Source: CAD feature listing. Evaluate the final solid. Frame: model axes, mm. Coordinates: 2 decimals unless noted, no trailing zeros. Loops run counter-clockwise (first coordinate to the right, second up) from the corner with the lowest first, then second, coordinate; pieces in that order, holes last.
Item 1: Section query B-B, the plane x = -62. Return the cut outline in (y, z), then the cut area to 3 significant figures.
Item 2: Pull-direction query (X, two-part tool) for faces 1 (the cylindrical face through (-20.652, 1.521, 32.192)), 2 (the flat face through (-7, 3, 38)), 3 (the cylindrical face through (60.413, 1.521, 38.969)); classes: +X half, -X half, draft (parallel to the pull), parting line (faces both ways), or undercut.
Item 3: Pin query (flat end, axial travel): pin 1 Ø2 at (x, z) = (-19.5, 38) entering from -Y. Return the tip coordinate at first contact, or that it passes through.
Item 4: Line query: probe 1 along Z at (x, y) = (-97.5, 1.8); probe 2 along Z at (x, y) = (-44, 0.85); probe 3 along Z at (x, y) = (15, 2.35). Output: solid intervals per line, ascending.
Item 5: Section query A-A, the plane z = 20. Return the cut outline in (x, y), then the cut area to 3 significant figures.
Item 6: Section query C-C, the plane y = 1.4. State how many separate pieces and enclosed holes the cut face has, then the cut area to 3 significant figures.
```python
from build123d import *

# Parameters (mm, degrees)
SKETCH1_W           = 214
SKETCH1_H           = 186
BOSS_EXTRUDE1_DEPTH = 3
SKETCH2_R           = 23
SPEAKER_DEPTH       = 4
SKETCH4_R           = 3
SKETCH4_R_2         = 1.025
MOTOR_DEPTH         = 4
SKETCH6_W           = 6
SKETCH6_H           = 5
IZGARALAR_DEPTH     = 4
SKETCH7_R           = 9.5
MOTOR_KABLOSU_DEPTH = 4


with BuildPart() as part:
    # Sketch1 → Boss-Extrude1 (new body)
    with BuildSketch(Plane(origin=(0, 0, 0), x_dir=(1, 0, 0), z_dir=(0, 1, 0))):
        with Locations((-5.589552239, -39.100746269)):
            Rectangle(SKETCH1_W, SKETCH1_H)
    extrude(amount=BOSS_EXTRUDE1_DEPTH)

    # Sketch2 → Speaker (cut, through all)
    with BuildSketch(Plane(origin=(0, 3, 0), x_dir=(1, 0, 0), z_dir=(0, 1, 0))):
        with Locations((-42.589552239, -39.100746269)):
            Circle(SKETCH2_R)
    extrude(amount=-SPEAKER_DEPTH, mode=Mode.SUBTRACT)

    # Sketch4 → Motor (cut, through all)
    with BuildSketch(Plane(origin=(0, 3, 0), x_dir=(1, 0, 0), z_dir=(0, 1, 0))):
        with Locations((63.410447761, -39.100746269)):
            Circle(SKETCH4_R)
        with Locations((63.410447761, -31.100746269)):
            Circle(SKETCH4_R_2)
        with Locations((71.410447761, -39.100746269)):
            Circle(SKETCH4_R_2)
        with Locations((63.410447761, -47.100746269)):
            Circle(SKETCH4_R_2)
        with Locations((55.410447761, -39.100746269)):
            Circle(SKETCH4_R_2)
    extrude(amount=-MOTOR_DEPTH, mode=Mode.SUBTRACT)

    # Sketch6 → Izgaralar (cut, through all)
    with BuildSketch(Plane(origin=(0, 3, 0), x_dir=(1, 0, 0), z_dir=(0, 1, 0))):
        with Locations((-97.589552239, -122.600746269)):
            Rectangle(SKETCH6_W, SKETCH6_H)
        with Locations((-50.589552239, -122.600746269)):
            Rectangle(SKETCH6_W, SKETCH6_H)
        with Locations((-3.589552239, -122.600746269)):
            Rectangle(SKETCH6_W, SKETCH6_H)
        with Locations((-97.589552239, 44.399253731)):
            Rectangle(SKETCH6_W, SKETCH6_H)
        with Locations((-50.589552239, 44.399253731)):
            Rectangle(SKETCH6_W, SKETCH6_H)
        with Locations((-3.589552239, 44.399253731)):
            Rectangle(SKETCH6_W, SKETCH6_H)
        with Locations((43.410447761, -122.600746269)):
            Rectangle(SKETCH6_W, SKETCH6_H)
        with Locations((43.410447761, 44.399253731)):
            Rectangle(SKETCH6_W, SKETCH6_H)
    extrude(amount=-IZGARALAR_DEPTH, mode=Mode.SUBTRACT)

    # Sketch7 → Motor Kablosu (cut, through all)
    with BuildSketch(Plane(origin=(0, 3, 0), x_dir=(1, 0, 0), z_dir=(0, 1, 0))):
        with Locations((6.410447761, -38.065571016)):
            Circle(SKETCH7_R)
    extrude(amount=-MOTOR_KABLOSU_DEPTH, mode=Mode.SUBTRACT)


solid = part.part
```
Verdict:
1. outline: (0, -53.9) - (3, -53.9) - (3, 26.76) - (0, 26.76) - close; (0, 51.44) - (3, 51.44) - (3, 132.1) - (0, 132.1) - close
1. area: 484 mm2
2. face 1: undercut
2. face 2: draft
2. face 3: undercut
3. pin 1: stops at y = 0
4. probe 1: z = -53.9 to -46.9, -41.9 to 120.1, 125.1 to 132.1
4. probe 2: z = -53.9 to 16.14, 62.06 to 132.1
4. probe 3: z = -53.9 to 34.01, 42.12 to 132.1
5. outline: (-112.59, 0) - (-55.4, 0) - (-55.4, 3) - (-112.59, 3) - close; (-29.78, 0) - (101.41, 0) - (101.41, 3) - (-29.78, 3) - close
5. area: 565 mm2
6. separate pieces: 1
6. enclosed holes: 15
6. area: 37,600 mm2
